Source: CAD feature listing. Evaluate the final solid. Frame: model axes, mm. Face numbers are marked on the shaded views. A direction names the side the tool comes from. Give positions to 0.01 mm unless a question says otherwise; leave off trailing zeros. Order: outer loops, then holes, each group sorted by start corner. A loop starts at its lowest first (then second) coordinate and runs counter-clockwise, first axis right, second up.
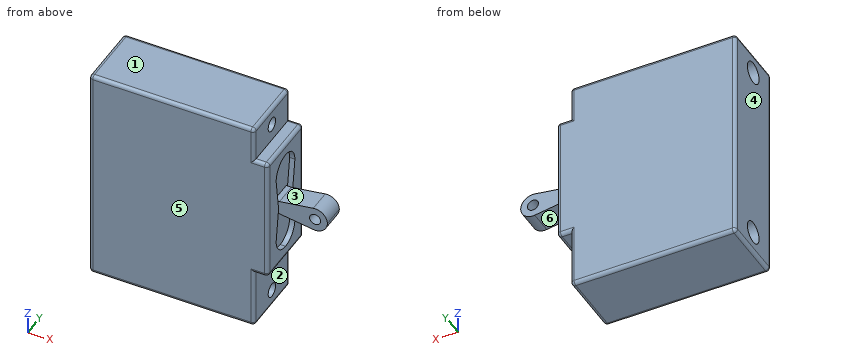
```python
from build123d import *

# Parameters (mm, degrees)
F0_W      = 47.2
F0_H      = 64
F1_DEPTH  = 9.5
F2_W      = 19
F2_H      = 36.6
F3_DEPTH  = 3.9
F5_DEPTH  = 1.5
F6_R      = 3.15
F7_DEPTH  = 8
F8_R      = 2
F9_DEPTH  = 4
F10_R     = 1.575
F11_DEPTH = 3.25
F12_R     = 1


with BuildPart() as f1:
    # F0 (on Front) → F1 (new body, symmetric)
    with BuildSketch(Plane.XZ):
        Rectangle(F0_W, F0_H)
    extrude(amount=F1_DEPTH, both=True)

    # F2 (on face) → F3 (join)
    with BuildSketch(Plane.YZ.offset(23.6)):
        with Locations((0, 3.7)):
            Rectangle(F2_W, F2_H)
    extrude(amount=F3_DEPTH)

    # F4 (on face) → F5 (cut)
    with BuildSketch(Plane.YZ.offset(27.5)):
        with BuildLine():
            ThreePointArc((3.865939, 3.030682), (3.820938, 3.7), (3.865939, 4.369318))
            Line((3.865939, 4.369318), (5.099388, 13.500612))
            ThreePointArc((5.099388, 13.500612), (3.605812, 17.106424), (0, 18.6))
            ThreePointArc((0, 18.6), (-3.605812, 17.106424), (-5.099388, 13.500612))
            Line((-5.099388, 13.500612), (-3.865939, 4.369318))
            ThreePointArc((-3.865939, 4.369318), (-3.820938, 3.7), (-3.865939, 3.030682))
            Line((-3.865939, 3.030682), (-5.099388, -6.100612))
            ThreePointArc((-5.099388, -6.100612), (-3.605812, -9.706424), (0, -11.2))
            ThreePointArc((0, -11.2), (3.605812, -9.706424), (5.099388, -6.100612))
            Line((5.099388, -6.100612), (3.865939, 3.030682))
        make_face()
    extrude(amount=-F5_DEPTH, mode=Mode.SUBTRACT)

    # F6 (on face) → F7 (cut)
    with BuildSketch(Plane(origin=(-23.6, 0, 0), x_dir=(0, -1, 0), z_dir=(-1, 0, 0))):
        with Locations((0, 26)):
            Circle(F6_R)
        with Locations((0, -26)):
            Circle(F6_R)
    extrude(amount=-F7_DEPTH, mode=Mode.SUBTRACT)

    # F8 (on face) → F9 (cut)
    with BuildSketch(Plane.YZ.offset(23.6)):
        with Locations((0, 27)):
            Circle(F8_R)
        with Locations((0, -27)):
            Circle(F8_R)
    extrude(amount=-F9_DEPTH, mode=Mode.SUBTRACT)

    # F10 (on Front) → F11 (join, symmetric)
    with BuildSketch(Plane.XZ):
        with BuildLine():
            ThreePointArc((37.146019, 0.239445), (39.952111, 1.046329), (41.17, 3.7))
            ThreePointArc((41.17, 3.7), (39.952111, 6.353671), (37.146019, 7.160555))
            ThreePointArc((37.146019, 7.160555), (34.17, 3.7), (37.146019, 0.239445))
        make_face()
        with Locations((37.67, 3.7)):
            Circle(F10_R, mode=Mode.SUBTRACT)
        with BuildLine():
            ThreePointArc((37.146019, 0.239445), (34.17, 3.7), (37.146019, 7.160555))
            Line((37.146019, 7.160555), (27.5, 5.7))
            Line((27.5, 5.7), (25.5, 5.7))
            Line((25.5, 5.7), (25.5, 1.7))
            Line((25.5, 1.7), (27.5, 1.7))
            Line((27.5, 1.7), (37.146019, 0.239445))
        make_face()
    extrude(amount=F11_DEPTH, both=True)

    # F12
    f12_edges = [f1.edges().sort_by_distance(p)[0] for p in [
        (0, 9.5, -32),
        (23.6, 9.5, -23.3),
        (25.55, 9.5, -14.6),
        (27.5, 9.5, 3.7),
        (25.55, 9.5, 22),
        (23.6, 9.5, 27),
        (0, 9.5, 32),
        (-23.6, 9.5, 0),
        (23.6, 0, 32),
        (-23.6, 0, 32),
        (0, -9.5, 32),
        (0, -9.5, -32),
        (23.6, -9.5, -23.3),
        (25.55, -9.5, -14.6),
        (27.5, -9.5, 3.7),
        (25.55, -9.5, 22),
        (23.6, -9.5, 27),
        (-23.6, -9.5, 0),
        (27.5, 0, -14.6),
        (27.5, 0, 22),
        (23.6, 0, -32),
        (-23.6, 0, -32),
    ]]
    fillet(f12_edges, radius=F12_R)


solid = f1.part
```
1) Draft query along X for the marked faces 3, 4, 5 and 6. Return one class per face: +X half, -X half, draft (parallel to the pull), parting line (faces both ways), or undercut.
Report:
face 3: undercut
face 4: -X half
face 5: draft
face 6: undercut
2) Pin query (flat end, axial travel): pin 1 (5.5 mm diameter, centred on x = 31.5, z = 3, fed in from +Y); pin 2 (3.5 mm diameter, centred on x = 36.5, z = 5.5, fed in from -Y); pin 3 (1.9 mm diameter, centred on y = 0.5, z = -26.5, fed in from -X). Return the tip coordinate at first contact, or that it passes through.
Report:
pin 1: stops at y = 3.25
pin 2: stops at y = -3.25
pin 3: stops at x = -15.6
3) Section query B-B, the plane z = -16. Return the cut outline in (x, y), and give its area (3 significant figures).
Report:
outline: (-23.6, -8.5) arc R1 ccw to (-22.6, -9.5) - (22.6, -9.5) arc R1 ccw to (23.6, -8.5) - (23.6, 8.5) arc R1 ccw to (22.6, 9.5) - (-22.6, 9.5) arc R1 ccw to (-23.6, 8.5) - close
area: 896 mm2
4) Reachability of the marked faces 1 and 2 from +Z, -Z, +X, -X, +Y, -Y: full face, straight path, thin tool, end or side. Return the list, or none.
Report:
face 1: +Z, +X, -X, +Y, -Y
face 2: -Z, +X, +Y, -Y
5) Material intervals for L1, parallel to Z at x = 21, y = 0; L2, parallel to Z at x = -19.25, y = 0; L3, parallel to X at y = -5.25, z = 1, sorted ascending.
Report:
L1: z = -32 to -29, -25 to 25, 29 to 32
L2: z = -32 to -29.15, -22.85 to 22.85, 29.15 to 32
L3: x = -23.6 to 27.5
6) Section query D-D, the plane x = 21.5. Return the cut outline in (y, z), and give its area (3 significant figures).
Report:
outline: (-9.5, -31) arc R1 ccw to (-8.5, -32) - (8.5, -32) arc R1 ccw to (9.5, -31) - (9.5, 31) arc R1 ccw to (8.5, 32) - (-8.5, 32) arc R1 ccw to (-9.5, 31) - close; hole circle Ø4 at (0, -27); hole circle Ø4 at (0, 27)
area: 1,190 mm2
7) Section query A-A, the plane x = -17. Return the cut outline in (y, z).
Report:
outline: (-9.5, -31) arc R1 ccw to (-8.5, -32) - (8.5, -32) arc R1 ccw to (9.5, -31) - (9.5, 31) arc R1 ccw to (8.5, 32) - (-8.5, 32) arc R1 ccw to (-9.5, 31) - close; hole circle Ø6.3 at (0, -26); hole circle Ø6.3 at (0, 26)
8) Section query C-C, the plane y = -7. Return the cut outline in (x, z).
Report:
outline: (-23.6, -31) arc R1 ccw to (-22.6, -32) - (22.6, -32) arc R1 ccw to (23.6, -31) - (23.6, -14.6) - (26.5, -14.6) arc R1 ccw to (27.5, -13.6) - (27.5, 21) arc R1 ccw to (26.5, 22) - (23.6, 22) - (23.6, 31) arc R1 ccw to (22.6, 32) - (-22.6, 32) arc R1 ccw to (-23.6, 31) - close
